```python
from build123d import *

# Parameters (mm, degrees)
PAD_DEPTH          = 10
SKETCH002_W        = 6
SKETCH002_H        = 8
POCKET_DEPTH       = 178.615176
POLARPATTERN_COUNT = 8
PAD001_DEPTH       = 2


with BuildPart() as part:
    # Sketch → Pad (new body)
    with BuildSketch(Plane.XY):
        with BuildLine():
            Line((-32, 7), (-32, -7))
            ThreePointArc((-32, -7), (-27.606602, -17.606602), (-17, -22))
            Line((-17, -22), (17, -22))
            ThreePointArc((17, -22), (27.606602, -17.606602), (32, -7))
            Line((32, -7), (32, 7))
            ThreePointArc((32, 7), (27.606602, 17.606602), (17, 22))
            Line((17, 22), (-17, 22))
            ThreePointArc((-17, 22), (-27.606602, 17.606602), (-32, 7))
        make_face()
        with BuildLine():
            Line((-30, 7), (-30, -7))
            ThreePointArc((-30, -7), (-26.192388, -16.192388), (-17, -20))
            Line((-17, -20), (17, -20))
            ThreePointArc((17, -20), (26.192388, -16.192388), (30, -7))
            Line((30, -7), (30, 7))
            ThreePointArc((30, 7), (26.192388, 16.192388), (17, 20))
            Line((17, 20), (-17, 20))
            ThreePointArc((-17, 20), (-26.192388, 16.192388), (-30, 7))
        make_face(mode=Mode.SUBTRACT)
    extrude(amount=PAD_DEPTH)

    # Sketch002 → Pocket (cut, through all)
    with BuildSketch(Plane.XZ):
        with Locations((0, 6)):
            Rectangle(SKETCH002_W, SKETCH002_H)
    pocket = extrude(amount=-POCKET_DEPTH, mode=Mode.SUBTRACT)

    # PolarPattern: Pocket ×8 about axis
    polarpattern_axis = Axis((0, 0, 0), (0, 0, 1))
    for i in range(1, POLARPATTERN_COUNT):
        add(pocket.rotate(polarpattern_axis, i * 360 / POLARPATTERN_COUNT), mode=Mode.SUBTRACT)

    # Sketch001 → Pad001 (join)
    with BuildSketch(Plane.XY):
        with BuildLine():
            Line((-31, 6), (-31, -6))
            ThreePointArc((-31, -6), (-26.606602, -16.606602), (-16, -21))
            Line((-16, -21), (16, -21))
            ThreePointArc((16, -21), (26.606602, -16.606602), (31, -6))
            Line((31, -6), (31, 6))
            ThreePointArc((31, 6), (26.606602, 16.606602), (16, 21))
            Line((16, 21), (-16, 21))
            ThreePointArc((-16, 21), (-26.606602, 16.606602), (-31, 6))
        make_face()
    extrude(amount=PAD001_DEPTH)


solid = part.part
```
Model file for the job. Use its own axes, mm. A direction names the side the tool comes from. Coordinates: 2 decimals unless noted, no trailing zeros. Order: outer loops, then holes, each group sorted by start corner. A loop starts at its lowest first (then second) coordinate and runs counter-clockwise, first axis right, second up. Notation, with made-up numbers: (-27.5, -28.75) -> (5.5, -28.75) arc R23 ccw to (5.5, -17.75) -> close; hole circle Ø8 at (45, -10). An arc over 180 degrees is marked (long way). Return JSON: item names as keys, results as strings.
Item 1: Wall check: line 1 along Y through (x, z) = (15, 6.5); line 2 along X through (y, z) = (-3.5, 9.75); line 3 along Z through (x, y) = (2, -7.5). Give the ranges that are in metal, low to high. Write a range as from..to.
Model answer:
{"line 1": "y = -22..-20, 20..22", "line 2": "x = -32..-30, 30..32", "line 3": "z = 0..2"}
Item 2: Slice it at C-C (y = -5). Write the cut outline in (x, z), then the cut area to 3 significant figures.
Model answer:
{"outline": "(-32, 0) -> (32, 0) -> (32, 10) -> (30, 10) -> (30, 2) -> (-30, 2) -> (-30, 10) -> (-32, 10) -> close", "area": "160 mm²"}
Item 3: Pin check, flat tips, straight feed: P1, Ø3, axis at y = 11, z = 7.5, coming from the -X side; P2, Ø0.6, axis at y = -21.5, z = 8, coming from the +X side; P3, Ø13, axis at x = -7, y = 4.5, coming from the +Z side. Stop position of each tip, or through.
Model answer:
{"P1": "stops at x = -31.79", "P2": "stops at x = 17.56", "P3": "stops at z = 2"}
Item 4: Slice it at A-A (x = 15). Write the cut outline in (y, z), then the cut area to 3 significant figures.
Model answer:
{"outline": "(-22, 0) -> (22, 0) -> (22, 10) -> (20, 10) -> (20, 2) -> (-20, 2) -> (-20, 10) -> (-22, 10) -> close", "area": "120 mm²"}
Item 5: Slice it at B-B (z = 4.75). Count the separate pieces of the cut face and the enclosed holes in it, then the cut area to 3 significant figures.
Model answer:
{"separate pieces": "8", "enclosed holes": "0", "area": "263 mm²"}
Item 6: Slice it at D-D (y = 1). Write the cut outline in (x, z).
Model answer:
{"outline": "(-32, 0) -> (32, 0) -> (32, 2) -> (-32, 2) -> close"}
Item 7: 3-axis set-ups, long thin cutter, end or side, ignore diameter. For faces 1 (the face through (-30, -5, 6)), 2 (the face through (-3, -21, 6)), 3 (the face through (-23.58, -19.34, 5.94)): which of +Z, -Z, +X, -X, +Y, -Y reach the whole face in a straight line?
Model answer:
{"face 1": "+Z", "face 2": "+Z, +Y, -Y", "face 3": "+Z, -Y"}
